The listing builds one solid part. Answer for the finished solid, in the listing's coordinates (mm). A direction names the side the tool comes from. Round coordinates to 2 decimals unless told otherwise and drop trailing zeros. Loops run counter-clockwise (first coordinate to the right, second up) from the corner with the lowest first, then second, coordinate; pieces in that order, holes last. Notation, with made-up numbers: (-18, 56.5) -> (18, 56.5) arc R12 cw to (18, 60.5) -> close; hole circle Ø2 at (-38, 29). An arc over 180 degrees is marked (long way). Use a Markdown table: item, result. Add a question column.
Q1. For a pull along Z with two mould halves and no side action, classify faces 4 (the cylindrical face through (9.46, 27.97, -0.07)), 5 (the cylindrical face through (-6.692, 27.972, 0.766)), 6 (the cylindrical face through (8.37, 27.97, -0.6)), 7 (the flat face through (-1, 30, 0)) as released by +Z, released by -Z, zero draft, split by the parting line, or undercut.
Q2. Section A-A on z = 0 is taken. Give the vertices of the cut face in (x, y), then the cut area to 3 significant figures.
Q3. Section C-C on x = -8 is taken. Give the vertices of the cut face in (y, z).
Q4. Given pin 1 Ø1.8 at (y, z) = (11.5, -1) entering from -X, flat-ended and moving along its own axis, determine where the tip first touches the part or whether it passes through.
Q5. Section D-D on y = 7.5 is taken. Give the vertices of the cut face in (x, z), then the cut area to 3 significant figures.
Q6. Consider line 1 (X direction, y = 2.65, z = 0); line 2 (Y direction, x = -6.5, z = 1.6); line 3 (X direction, y = 1.75, z = 1.35). Determine where each line is inside the solid, lowest interval first.
Q7. Section B-B on x = 7.5 is taken. Give the vertices of the cut face in (y, z), then the cut area to 3 significant figures.
Q8. Which of the six approach directions +Z, -Z, +X, -X, +Y, -Y give full straight-line access (tool end or side, diameter ignored) to faces 1 (the cylindrical face through (-11.54, 27.97, 0.07)), 2 (the flat face through (4, 4, 0)), 3 (the flat face through (-6.5, 4, 0.7))?
from build123d import *

# Parameters (mm, degrees)
SKETCH1_R           = 2
BOSS_EXTRUDE1_DEPTH = 30
CUT_EXTRUDE1_REACH  = 8
SKETCH3_W           = 7
SKETCH3_H           = 22


with BuildPart() as part:
    # Sketch1 → Boss-Extrude1 (new body)
    with BuildSketch(Plane(origin=(0, 0, 0), x_dir=(1, 0, 0), z_dir=(0, 1, 0))):
        with BuildLine():
            Line((-8.539325843, 3), (6.460674157, 3))
            ThreePointArc((6.460674157, 3), (9.460674157, 0), (6.460674157, -3))
            Line((6.460674157, -3), (-8.539325843, -3))
            ThreePointArc((-8.539325843, -3), (-11.539325843, 0), (-8.539325843, 3))
        make_face()
        with Locations((-8.539325843, 0)):
            Circle(SKETCH1_R, mode=Mode.SUBTRACT)
        with Locations((6.460674157, 0)):
            Circle(SKETCH1_R, mode=Mode.SUBTRACT)
    extrude(amount=BOSS_EXTRUDE1_DEPTH)

    # Sketch3 → Cut-Extrude1 (cut, up to next)
    with BuildSketch(Plane.XY.offset(3), mode=Mode.PRIVATE) as cut_extrude1_sk1:
        with Locations((5.960674157, 15)):
            Rectangle(SKETCH3_W, SKETCH3_H)
    cut_extrude1_tool1 = extrude(cut_extrude1_sk1.sketch, amount=-CUT_EXTRUDE1_REACH, mode=Mode.PRIVATE) & part.part
    add(cut_extrude1_tool1.solids().sort_by_distance((5.960674, 15, 3))[0], mode=Mode.SUBTRACT)
    # Sketch3 → Cut-Extrude1 (cut, up to next)
    with BuildSketch(Plane.XY.offset(3), mode=Mode.PRIVATE) as cut_extrude1_sk2:
        with Locations((-8.039325843, 15)):
            Rectangle(SKETCH3_W, SKETCH3_H)
    cut_extrude1_tool2 = extrude(cut_extrude1_sk2.sketch, amount=-CUT_EXTRUDE1_REACH, mode=Mode.PRIVATE) & part.part
    add(cut_extrude1_tool2.solids().sort_by_distance((-8.039326, 15, 3))[0], mode=Mode.SUBTRACT)


solid = part.part
Checked values:
| question | item | result |
|---|---|---|
| 1 | face 4 | split by the parting line |
| 1 | face 5 | undercut |
| 1 | face 6 | undercut |
| 1 | face 7 | zero draft |
| 2 | outline | (-11.54, 0) -> (-10.54, 0) -> (-10.54, 4) -> (-11.54, 4) -> close; (-11.54, 26) -> (-10.54, 26) -> (-10.54, 30) -> (-11.54, 30) -> close; (-6.54, 0) -> (4.46, 0) -> (4.46, 4) -> (2.46, 4) -> (2.46, 26) -> (4.46, 26) -> (4.46, 30) -> (-6.54, 30) -> (-6.54, 26) -> (-4.54, 26) -> (-4.54, 4) -> (-6.54, 4) -> close; (8.46, 0) -> (9.46, 0) -> (9.46, 4) -> (8.46, 4) -> close; (8.46, 26) -> (9.46, 26) -> (9.46, 30) -> (8.46, 30) -> close |
| 2 | area | 258 mm2 |
| 3 | outline | (0, -3) -> (4, -3) -> (4, -1.93) -> (0, -1.93) -> close; (0, 1.93) -> (4, 1.93) -> (4, 3) -> (0, 3) -> close; (26, -3) -> (30, -3) -> (30, -1.93) -> (26, -1.93) -> close; (26, 1.93) -> (30, 1.93) -> (30, 3) -> (26, 3) -> close |
| 4 | pin 1 | stops at x = -4.54 |
| 5 | outline | (-4.54, -3) -> (2.46, -3) -> (2.46, 3) -> (-4.54, 3) -> close |
| 5 | area | 42.0 mm2 |
| 6 | line 1 | x = -11.54 to -10.54, -6.54 to 4.46, 8.46 to 9.46 |
| 6 | line 2 | y = 0 to 4, 26 to 30 |
| 6 | line 3 | x = -11.22 to -10.01, -7.06 to 4.99, 7.94 to 9.14 |
| 7 | outline | (0, -2.81) -> (4, -2.81) -> (4, -1.71) -> (0, -1.71) -> close; (0, 1.71) -> (4, 1.71) -> (4, 2.81) -> (0, 2.81) -> close; (26, -2.81) -> (30, -2.81) -> (30, -1.71) -> (26, -1.71) -> close; (26, 1.71) -> (30, 1.71) -> (30, 2.81) -> (26, 2.81) -> close |
| 7 | area | 17.7 mm2 |
| 8 | face 1 | -X, +Y, -Y |
| 8 | face 2 | +Z, -Z, +X |
| 8 | face 3 | +Z, -Z, -X |
